Geometry check sheet. Reference: the model listing, model coordinates, mm. A direction names the side the tool comes from. Give positions to 0.01 mm unless a question says otherwise; leave off trailing zeros. Order: outer loops, then holes, each group sorted by start corner. A loop starts at its lowest first (then second) coordinate and runs counter-clockwise, first axis right, second up.
from build123d import *

# Parameters (mm, degrees)
SKETCH1_W                    = 179.07
SKETCH1_H                    = 89.916
BOSS_EXTRUDE1_DEPTH          = 3.0734
F_30_0_1285_DIAMETER_HOLE1_D = 3.2639
F_30_0_1285_DIAMETER_HOLE2_D = 3.2639
SKETCH6_W                    = 15.24
SKETCH6_H                    = 60.96
SKETCH6_W_2                  = 135.89
SKETCH6_H_2                  = 10.16
CUT_EXTRUDE1_DEPTH           = 4.0734
FILLET2_R                    = 2.54


with BuildPart() as part:
    # Sketch1 → Boss-Extrude1 (new body)
    with BuildSketch(Plane(origin=(0, 0, 0), x_dir=(1, 0, 0), z_dir=(0, 1, 0))):
        Rectangle(SKETCH1_W, SKETCH1_H)
    extrude(amount=BOSS_EXTRUDE1_DEPTH)

    # #30 (0.1285) Diameter Hole1 (through all)
    with Locations(Plane(origin=(0, 3.0734, 0), x_dir=(1, 0, 0), z_dir=(0, 1, 0))):
        with Locations((-85.725, 41.021), (-85.725, -41.021), (85.725, -41.021), (85.725, 41.021)):
            Hole(F_30_0_1285_DIAMETER_HOLE1_D / 2)

    # #30 (0.1285) Diameter Hole2 (through all)
    with Locations(Plane(origin=(0, 3.0734, 0), x_dir=(1, 0, 0), z_dir=(0, 1, 0))):
        with Locations((-0.215, 24.5), (-0.215, -24.5), (57.785, -24.5), (57.785, 24.5)):
            Hole(F_30_0_1285_DIAMETER_HOLE2_D / 2)

    # Sketch6 → Cut-Extrude1 (cut, through all)
    with BuildSketch(Plane(origin=(0, 3.0734, 0), x_dir=(1, 0, 0), z_dir=(0, 1, 0))):
        with Locations((-81.915, 0)):
            Rectangle(SKETCH6_W, SKETCH6_H)
        with Locations((13.97, -39.878)):
            Rectangle(SKETCH6_W_2, SKETCH6_H_2)
        with Locations((13.97, 39.878)):
            Rectangle(SKETCH6_W_2, SKETCH6_H_2)
    extrude(amount=-CUT_EXTRUDE1_DEPTH, mode=Mode.SUBTRACT)

    # Fillet2
    fillet2_edges = [part.edges().sort_by_distance(p)[0] for p in [
        (-89.535, 1.5367, 30.48),
        (-89.535, 1.5367, -30.48),
        (-74.295, 1.5367, -30.48),
        (-74.295, 1.5367, 30.48),
        (-89.535, 1.5367, -44.958),
        (89.535, 1.5367, -44.958),
        (89.535, 1.5367, 44.958),
        (-89.535, 1.5367, 44.958),
        (-53.975, 1.5367, 44.958),
        (-53.975, 1.5367, 34.798),
        (81.915, 1.5367, 34.798),
        (81.915, 1.5367, 44.958),
        (-53.975, 1.5367, -34.798),
        (-53.975, 1.5367, -44.958),
        (81.915, 1.5367, -44.958),
        (81.915, 1.5367, -34.798),
    ]]
    fillet(fillet2_edges, radius=FILLET2_R)


solid = part.part
Item 1: Draft check along X on faces 1 (the flat face through (-89.535, 2, -38)), 2 (the flat face through (-1, 0, -1)), 3 (the flat face through (13, 2, 34.798)). Enter one of: released by +X, released by -X, zero draft, split by the parting line, or undercut.
Reported:
face 1: released by -X
face 2: zero draft
face 3: undercut
Item 2: Sectioned sample at B-B (x = 43.5). Enter the section's corners in (y, z), and give its area (3 significant figures).
Reported:
outline: (0, -34.8) - (3.07, -34.8) - (3.07, 34.8) - (0, 34.8) - close
area: 214 mm2
Item 3: Sectioned sample at A-A (z = 24.5). Enter the section's corners in (x, y) (3 decimals).
Reported:
outline: (-74.295, 0) - (-1.847, 0) - (-1.847, 3.073) - (-74.295, 3.073) - close; (1.417, 0) - (56.153, 0) - (56.153, 3.073) - (1.417, 3.073) - close; (59.417, 0) - (89.535, 0) - (89.535, 3.073) - (59.417, 3.073) - close
Item 4: Set-up check for faces 4 (the flat face through (-82, 2, 30.48)), 5 (the flat face through (81.915, 2, 40)), 6 (the flat face through (13, 2, -34.798)), 7 (the cylindrical face through (-86.48, 1.52, 42.47)): record each of +Z, -Z, +X, -X, +Y, -Y from which the full face is reachable in a straight line by a thin tool's end or side.
Reported:
face 4: -X, +Y, -Y
face 5: +Z, +Y, -Y
face 6: -Z, +Y, -Y
face 7: +Y, -Y
Item 5: Gauge pin test, flat ends, axial feed: pin 1 (1.5 mm diameter, centred on y = 2, z = -21.5, fed in from -X) (3 decimals); pin 2 (0.9 mm diameter, centred on x = -5.5, y = 2, fed in from -Z); pin 3 (1.5 mm diameter, centred on x = 31, y = 1, fed in from +Z). Record the tip position at first contact, or that the pin passes through.
Reported:
pin 1: stops at x = -74.295
pin 2: stops at z = -34.8
pin 3: stops at z = 34.8
Item 6: Scan lines: L1, parallel to Z at x = 57, y = 1.3; L2, parallel to X at y = 2.2, z = -40 (3 decimals); L3, parallel to X at y = 2.45, z = 5.5 (3 decimals). Record each from-to range of solid material in increasing order.
Reported:
L1: z = -34.8 to -25.93, -23.07 to 23.07, 25.93 to 34.8
L2: x = -89.535 to -86.998, -84.452 to -53.975, 81.915 to 84.452, 86.998 to 89.535
L3: x = -74.295 to 89.535
Item 7: Sectioned sample at C-C (y = 0.65). Give the number of separate pieces and of enclosed holes in the cut face, and give its area (3 significant figures).
Reported:
separate pieces: 1
enclosed holes: 8
area: 12,300 mm2
